Build history of the part. All positions in model axes, mm. A direction names the side the tool comes from. Round coordinates to 2 decimals unless told otherwise and drop trailing zeros. Write each loop counter-clockwise with the first axis right and the second up, starting at its lowest first coordinate (ties: lowest second). Pieces come first, ordered by that corner, then holes. Notation, with made-up numbers: M 27.25,63 L 68.25,63 A17 ccw 68.25,90 Z; hole C -1.5,-23 d4. An arc over 180 degrees is marked long. One line per item, written item: value. Start each with the question number.
Autodesk Inventor part; units mm, degrees
ref_plane "YZ Plane" through (0, 0, 0) normal (1, 0, 0) x (0, 1, 0)
ref_plane "XZ Plane" through (0, 0, 0) normal (0, 1, 0) x (-1, 0, 0)
ref_plane "XY Plane" through (0, 0, 0) normal (0, 0, 1) x (1, 0, 0)
sketch "Sketch1" plane through (0, 0, 0) normal (0, 1, 0) x (-1, 0, 0)
  line L0 (23, -43.5) -> (23, -56.5)
  line L1 (28, -33.25) -> (23, -33.25)
  line L2 (28, -30.75) -> (23, -30.75)
  line L3 (28, -48.75) -> (23, -48.75)
  line L4 (10, -56.5) -> (23, -56.5)
  line L5 (10, -7.5) -> (10, -20.5)
  line L6 (23, -43.5) -> (10, -43.5)
  line L7 (10, -43.5) -> (10, -56.5)
  line L8 (10, -38.5) -> (23, -38.5)
  line L9 (23, -38.5) -> (23, -25.5)
  line L10 (25.5, 0.6818) -> (25.5, -55.6748) construction
  line L11 (16.5, 0.1481) -> (16.5, -50.7513) construction
  line L12 (10, -25.5) -> (10, -38.5)
  line L13 (32.1467, -32) -> (-0.6768, -32) construction
  line L14 (10, -20.5) -> (23, -20.5)
  line L15 (23, -25.5) -> (10, -25.5)
  line L16 (23, -7.5) -> (10, -7.5)
  line L17 (30.1668, -14) -> (1.95, -14) construction
  line L18 (1.5, -34.25) -> (10, -34.25)
  line L19 (1.6727, -50) -> (31.8542, -50) construction
  line L20 (28, -60) -> (0, -60)
  line L21 (23, -51.25) -> (28, -51.25)
  line L22 (23, -7.5) -> (23, -20.5)
  line L23 (0, -29.75) -> (10, -29.75)
  line L24 (23, -15.25) -> (28, -15.25)
  line L25 (23, -12.75) -> (28, -12.75)
  line L26 (1.5, -16.25) -> (10, -16.25)
  line L27 (0, -11.75) -> (10, -11.75)
  line L28 (0, -47.75) -> (10, -47.75)
  line L29 (1.5, -52.25) -> (10, -52.25)
  line L30 (28, 0) -> (0, 0)
  line L31 (28, 0) -> (32, 0)
  line L32 (32, 0) -> (32, -66)
  line L33 (32, -66) -> (-4, -66)
  line L34 (-4, -66) -> (-4, 0)
  line L35 (28, -5) -> (30, -5)
  line L36 (30, -5) -> (30, -50)
  line L37 (30, -50) -> (32, -50)
  line L38 (-4, 0) -> (0, 0)
  line L39 (0, -5) -> (-2, -5)
  line L40 (-2, -5) -> (-2, -64)
  line L41 (-2, -64) -> (32, -64)
  line L42 (28, -4) -> (0, -4)
  line L43 (38, -5) -> (-10, -5) construction
  line L44 (0, -60) -> (0, -55.25)
  line L45 (0, -47.75) -> (0, -37.25)
  line L46 (0, -29.75) -> (0, -19.25)
  line L47 (0, -11.75) -> (0, 0)
  line L48 (1.5, -11.75) -> (1.5, -16.25)
  line L49 (1.5, -29.75) -> (1.5, -34.25)
  line L50 (1.5, -47.75) -> (1.5, -52.25)
  line L51 (1.5, -52.25) -> (1.5, -55.25)
  line L52 (1.5, -55.25) -> (0, -55.25)
  line L53 (1.5, -34.25) -> (1.5, -37.25)
  line L54 (1.5, -37.25) -> (0, -37.25)
  line L55 (1.5, -16.25) -> (1.5, -19.25)
  line L56 (1.5, -19.25) -> (0, -19.25)
  line L57 (28, 0) -> (28, -5)
  line L58 (31, -55.625) -> (29, -55.625) construction
  line L59 (28, -53.625) -> (26.5, -53.625)
  line L60 (26.5, -53.625) -> (26.5, -57.625)
  line L61 (26.5, -57.625) -> (28, -57.625)
  line L62 (28, -5) -> (28, -53.625)
  line L63 (28, -57.625) -> (28, -60)
  point P0 (16.5, -14)
  point P1 (16.5, -32)
  point P2 (16.5, -50)
  dimension "d0" = 13
  dimension "d3" = 2.5
  dimension "d6" = 4.5
  dimension "d7" = 4.5
  dimension "d8" = 4.5
  dimension "d10" = 13
  dimension "d11" = 18
  dimension "d12" = 18
  dimension "d13" = 13
  dimension "d16" = 13
  dimension "d17" = 3.5
  dimension "d18" = 4
  dimension "d20" = 45
  dimension "d21" = 4
  dimension "d22" = 2
  dimension "d23" = 2.5
  dimension "d24" = 3.5
  dimension "d25" = 4
  dimension "d26" = 2.5
  dimension "d27" = 2
  dimension "d28" = 4
  dimension "d29" = 66
  dimension "d30" = 36
  dimension "d37" = 1.5
  dimension "d38" = 10
  dimension "d39" = 2.5
  dimension "d55" = 3
  dimension "d58" = 28
  dimension "d59" = 2
  dimension "d60" = 1.5
  dimension "d61" = 4
extrude "Extrusion1" add sketch "Sketch1" against normal blind 2 contours L57 L31 L32 L37 L36 L35 | L42 L47 L30 L57 | L47 L39 L40 L41 L32 L33 L34 L38
extrude "Extrusion4" add sketch "Sketch1" against normal blind 7.5 contours L3 L62 L21 L0 | L7 L29 L50 L28 | L1 L9 L2 L62 | L24 L22 L25 L62 | L18 L49 L23 L12 | L26 L48 L27 L5
extrude "Extrusion5" add sketch "Sketch1" against normal blind 5 contours L6 L7 L28 L45 L54 L53 L18 L12 L8 L9 L1 L62 L3 L0 | L21 L62 L59 L60 L61 L63 L20 L44 L52 L51 L29 L7 L4 L0 | L2 L9 L15 L12 L23 L46 L56 L55 L26 L5 L14 L22 L24 L62 | L25 L22 L16 L5 L27 L47 L42 L57 L62
extrude "Extrusion6" add sketch "Sketch1" along normal blind 5 contours L6 L7 L28 L45 L54 L53 L18 L12 L8 L9 L1 L62 L3 L0 | L3 L62 L21 L0 | L21 L62 L59 L60 L61 L63 L20 L44 L52 L51 L29 L7 L4 L0 | L62 L35 L36 L37 L32 L41 L40 L39 L47 L27 L48 L55 L56 L46 L23 L49 L53 L54 L45 L28 L50 L51 L52 L44 L20 L63 L61 L60 L59 | L7 L29 L50 L28 | L1 L9 L2 L62 | L2 L9 L15 L12 L23 L46 L56 L55 L26 L5 L14 L22 L24 L62 | L24 L22 L25 L62 | L25 L22 L16 L5 L27 L47 L42 L57 L62 | L18 L49 L23 L12 | L57 L31 L32 L37 L36 L35 | L42 L47 L30 L57 | L26 L48 L27 L5 | L47 L39 L40 L41 L32 L33 L34 L38
sketch "Sketch2" plane through (0, 5, 0) normal (0, 1, 0) x (1, 0, 0)
  line L0 (-25, 3) -> (-3, 3)
  line L1 (1, 7) -> (1, 57)
  line L2 (-3, 61) -> (-25, 61)
  line L3 (-29, 57) -> (-29, 7)
  line L4 (-32, 66) -> (-32, 0)
  line L5 (-32, 0) -> (4, 0)
  line L6 (4, 0) -> (4, 66)
  line L7 (4, 66) -> (-32, 66)
  arc A0 (-29, 7) -> (-25, 3) centre (-25, 7) ccw
  arc A1 (-25, 61) -> (-29, 57) centre (-25, 57) ccw
  arc A2 (-3, 3) -> (1, 7) centre (-3, 7) ccw
  arc A3 (1, 57) -> (-3, 61) centre (-3, 57) ccw
  point P0 (0, 0)
  dimension "d46" = 3
  dimension "d47" = 3
  dimension "d48" = 3
  dimension "d49" = 5
  dimension "d54" = 8
extrude "Extrusion7" add sketch "Sketch2" along normal blind 3 contours A0 L3 A1 L2 A3 L1 A2 L0
extrude "Extrusion8" cut sketch "Sketch1" along normal blind 10 contours L0 L4 L7 L6 | L9 L8 L12 L15 | L22 L14 L5 L16
properties part number "Top_V3"
Item 1: Cut at D-D, the plane x = -24. Write the cut outline in (y, z), plus the area to 3 significant figures.
Item 2: Cut at A-A, the plane z = -31.5. Write the cut outline in (x, y).
Item 3: Which spindle directions (+Z, -Z, +X, -X, +Y, -Y) get a long thin tool onto all of the face, cutting with end or side? Do faces 1 (the flat face through (-23, 2, -14)), 2 (the flat face through (2, -1, -34)), 3 (the flat face through (-26, -6, -33.25)). Say none if no direction does.
Item 4: Two-plate mould, pull along X, no slides. Class faces 4 (the flat face through (-14, 2, -66)), 5 (the cylindrical face through (-0.141, 6.479, -4.203)), 6 (the flat face through (0, -2, -25)), 7 (the flat face through (-1, -2, -37.25)): pulls with the +X half, pulls with the -X half, needs draft (parallel to the pull), parting line crosses it, or undercut.
Item 5: Drill centre lines: line 1 (Z direction, x = -22, y = 6); line 2 (X direction, y = -5.75, z = -32); line 3 (Z direction, x = -29, y = -0.75). Where is each one in solid material? Low to high.
Item 6: Cut at C-C, the plane x = -11.5. Write the cut outline in (y, z).
Item 7: Cut at B-B, the plane y = -3. Count the separate pieces of the cut face and the enclosed holes in it, plus the area to 3 significant figures.
Item 8: Drop flat-ended pins along their axis: pin 1 (0.8 mm diameter, centred on x = -25, y = -5.5, fed in from +Z); pin 2 (1.2 mm diameter, centred on x = -7.5, y = -6, fed in from -Z); pin 3 (0.8 mm diameter, centred on x = -6, y = -6, fed in from +Z). Give the stop position or say it passes through.
Computed values:
1. outline: M -7.5,-51.25 L -5,-51.25 L -5,-60 L 0,-60 L 0,-64 L -2,-64 L -2,-66 L 5,-66 L 5,-61 L 8,-61 L 8,-3 L 5,-3 L 5,0 L -2,0 L -2,-4 L -5,-4 L -5,-12.75 L -7.5,-12.75 L -7.5,-15.25 L -5,-15.25 L -5,-30.75 L -7.5,-30.75 L -7.5,-33.25 L -5,-33.25 L -5,-48.75 L -7.5,-48.75 Z
1. area: 815 mm2
2. outline: M -32,-2 L -30,-2 L -30,0 L -28,0 L -28,-7.5 L -23,-7.5 L -23,8 L -29,8 L -29,5 L -32,5 Z; M -10,-7.5 L -1.5,-7.5 L -1.5,0 L 2,0 L 2,-2 L 4,-2 L 4,5 L 1,5 L 1,8 L -10,8 Z
3. face 1: +Y, -Y
3. face 2: -Y
3. face 3: -X, -Y
4. face 4: needs draft
4. face 5: pulls with the +X half
4. face 6: undercut
4. face 7: undercut
5. line 1: z = -61 to -56.5, -43.5 to -38.5, -25.5 to -20.5, -7.5 to -3
5. line 2: x = -28 to -23, -10 to -1.5
5. line 3: z = -66 to -64, -5 to 0
6. outline: M -5,-60 L 0,-60 L 0,-64 L -2,-64 L -2,-66 L 5,-66 L 5,-61 L 8,-61 L 8,-56.5 L -5,-56.5 Z; M -5,-43.5 L 8,-43.5 L 8,-38.5 L -5,-38.5 Z; M -5,-25.5 L 8,-25.5 L 8,-20.5 L -5,-20.5 Z; M -5,-7.5 L 8,-7.5 L 8,-3 L 5,-3 L 5,0 L -2,0 L -2,-4 L -5,-4 Z
7. separate pieces: 1
7. enclosed holes: 3
7. area: 1,020 mm2
8. pin 1: stops at z = -12.75
8. pin 2: stops at z = -52.25
8. pin 3: stops at z = -11.75
